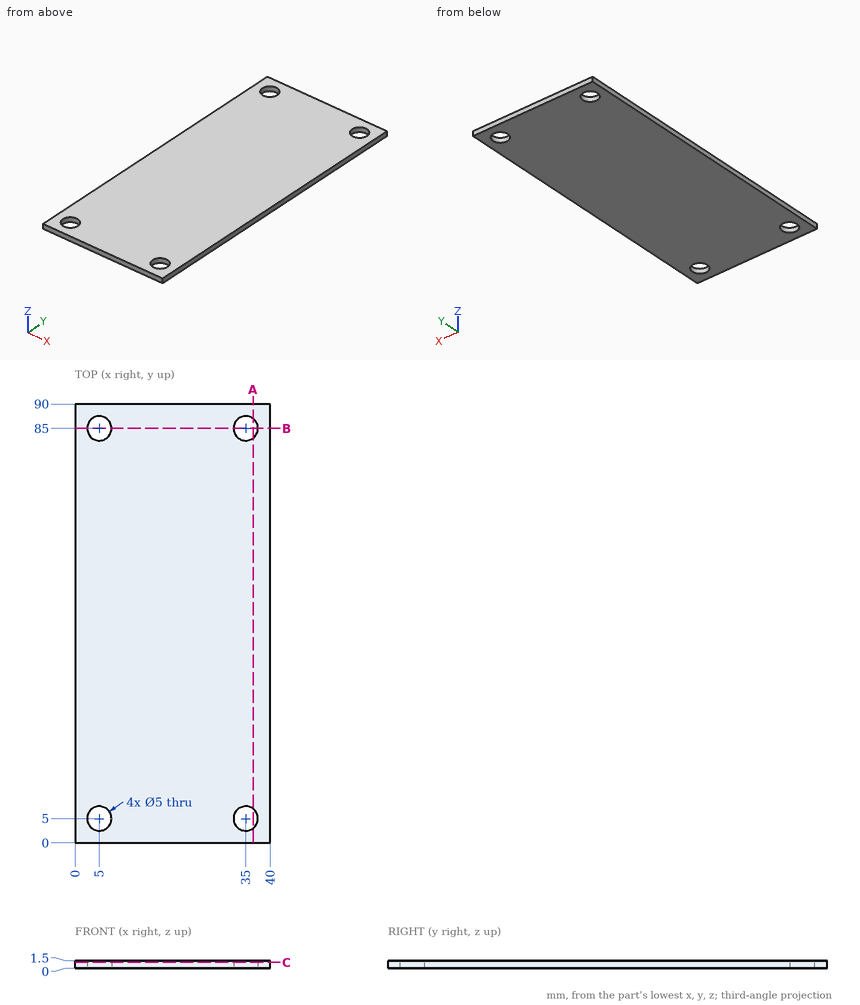
Design review of the part shown in the three views and the two pictorial views. Dimensions are in mm from the part's minimum x, y and z. Give positions to 0.01 mm unless a question says otherwise; leave off trailing zeros. Loops run counter-clockwise (first coordinate to the right, second up) from the corner with the lowest first, then second, coordinate; pieces in that order, holes last. Notation, with made-up numbers: (20, 48.25) -> (26, 48.25) arc R24 cw to (26, 69.25) -> close; hole circle Ø1 at (89, 15). An arc over 180 degrees is marked (long way). Answer as a JSON object with one key per item and string values. Group by question number.
Q1. Take a section at C-C (z = 1.2). Write out the cut boundary in (x, y).
Q2. Take a section at A-A (x = 36.5). Write out the cut boundary in (y, z), plus the area to 3 significant figures.
Q3. Take a section at B-B (y = 85). Write out the cut boundary in (x, z), plus the area to 3 significant figures.
Q4. Wall thickness on line 1 along X through (y, z) = (85, 0.5); line 2 along Y through (x, z) = (5, 0.4); line 3 along Y through (x, z) = (36, 0.25): over which ranges is each line inside the solid? List them lowest first.
Answer below:
{
 "1": {"outline": "(0, 0) -> (40, 0) -> (40, 90) -> (0, 90) -> close; hole circle Ø5 at (5, 5); hole circle Ø5 at (5, 85); hole circle Ø5 at (35, 5); hole circle Ø5 at (35, 85)"},
 "2": {"outline": "(0, 0) -> (3, 0) -> (3, 1.5) -> (0, 1.5) -> close; (7, 0) -> (83, 0) -> (83, 1.5) -> (7, 1.5) -> close; (87, 0) -> (90, 0) -> (90, 1.5) -> (87, 1.5) -> close", "area": "123 mm2"},
 "3": {"outline": "(0, 0) -> (2.5, 0) -> (2.5, 1.5) -> (0, 1.5) -> close; (7.5, 0) -> (32.5, 0) -> (32.5, 1.5) -> (7.5, 1.5) -> close; (37.5, 0) -> (40, 0) -> (40, 1.5) -> (37.5, 1.5) -> close", "area": "45.0 mm2"},
 "4": {"line 1": "x = 0 to 2.5, 7.5 to 32.5, 37.5 to 40", "line 2": "y = 0 to 2.5, 7.5 to 82.5, 87.5 to 90", "line 3": "y = 0 to 2.71, 7.29 to 82.71, 87.29 to 90"}
}
